Part model, mm, in its own coordinate system. Face numbers are marked on the shaded views. A direction names the side the tool comes from. Coordinates: 2 decimals unless noted, no trailing zeros. Loops run counter-clockwise (first coordinate to the right, second up) from the corner with the lowest first, then second, coordinate; pieces in that order, holes last. Notation, with made-up numbers: M -23,25 L 30,25 A32 ccw 30,62 Z; hole C 8.5,-38.5 d10. An arc over 180 degrees is marked long. Answer as CSV lines item,"result". Start each with the question number.
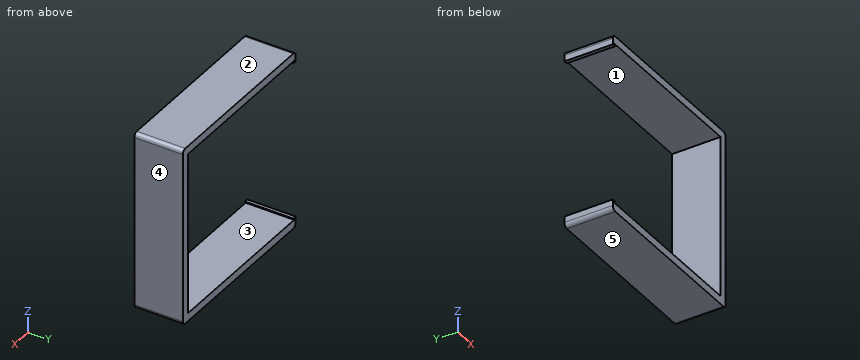
from build123d import *

# Parameters (mm, degrees)
F1_DEPTH = 12


with BuildPart() as f1:
    # F0 (on Front) → F1 (new body)
    with BuildSketch(Plane.XZ):
        with BuildLine():
            Line((-20, 20), (20, 20))
            Line((20, 20), (20, -20))
            Line((20, -20), (-20, -20))
            Line((-20, -20), (-21.379289, -20))
            ThreePointArc((-21.379289, -20), (-21.425483, -19.969134), (-21.414645, -19.914645))
            Line((-21.414645, -19.914645), (-21.085355, -19.585355))
            ThreePointArc((-21.085355, -19.585355), (-21.074517, -19.530866), (-21.120711, -19.5))
            Line((-21.120711, -19.5), (-22, -19.5))
            Line((-22, -19.5), (-22, -21))
            ThreePointArc((-22, -21), (-21.707107, -21.707107), (-21, -22))
            Line((-21, -22), (21, -22))
            ThreePointArc((21, -22), (21.707107, -21.707107), (22, -21))
            Line((22, -21), (22, 21))
            ThreePointArc((22, 21), (21.707107, 21.707107), (21, 22))
            Line((21, 22), (-21, 22))
            ThreePointArc((-21, 22), (-21.707107, 21.707107), (-22, 21))
            Line((-22, 21), (-22, 19.5))
            Line((-22, 19.5), (-21.133234, 19.5))
            ThreePointArc((-21.133234, 19.5), (-21.082247, 19.534068), (-21.094211, 19.594211))
            Line((-21.094211, 19.594211), (-21.5, 20))
            Line((-21.5, 20), (-20, 20))
        make_face()
    extrude(amount=F1_DEPTH)


solid = f1.part
Q1. Slice it at C-C, the plane z = 0. Write the cut outline in (x, y).
Q2. Slice it at A-A, the plane x = 17. Write the cut outline in (y, z), and give its area (3 significant figures).
Q3. Wall check: L1, parallel to Z at x = 14.5, y = -5.75; L2, parallel to X at y = -6.5, z = 16. Give the ranges that are in metal, low to high.
Q4. Tool access for the marked faces 1 and 2: list every direction of +Z, -Z, +X, -X, +Y, -Y with a clear straight run to the whole face (end or side of a thin tool).
Q5. Two-plate mould, pull along X, no slides. Class the marked faces 3, 4 and 5: +X half, -X half, draft (parallel to the pull), parting line (faces both ways), or undercut.
Q6. Flat gauge pin, fed straight in: P1, Ø0.7, axis at x = -21.5, y = -5, coming from the -Z side. Where does the tip first touch, or does it go through?
Q7. Slice it at B-B, the plane y = -1.25. Write the cut outline in (x, z), and give its area (3 significant figures).
Solved:
1,outline,"M 20,-12 L 22,-12 L 22,0 L 20,0 Z"
2,outline,"M -12,-22 L 0,-22 L 0,-20 L -12,-20 Z; M -12,20 L 0,20 L 0,22 L -12,22 Z"
2,area,"48.0 mm2"
3,L1,"z = -22 to -20, 20 to 22"
3,L2,"x = 20 to 22"
4,face 1,"+Y, -Y"
4,face 2,"+Z, +X, -X, +Y, -Y"
5,face 3,"undercut"
5,face 4,"+X half"
5,face 5,"draft"
6,P1,"stops at z = -21.99"
7,outline,"M -22,-21 A1 ccw -21,-22 L 21,-22 A1 ccw 22,-21 L 22,21 A1 ccw 21,22 L -21,22 A1 ccw -22,21 L -22,19.5 L -21.13,19.5 A0.06 ccw -21.09,19.59 L -21.5,20 L 20,20 L 20,-20 L -21.38,-20 A0.05 cw -21.41,-19.91 L -21.09,-19.59 A0.05 ccw -21.12,-19.5 L -22,-19.5 Z"
7,area,"256 mm2"
